Read the model definition and answer for the solid it produces. Units are mm, in the model's axes. Coordinates: 2 decimals unless noted, no trailing zeros.
1) Determine the mould class of faces 1 (the face through (-0.66, -14.985, 25.35)), 2 (the face through (4, -16, 0)) for opening direction X: +X half, -X half, draft (parallel to the pull), parting line (faces both ways), or undercut.
2) Each of these flat-tipped pins is pushed along its axis until it touches: pin 1 Ø2 at (y, z) = (-28.5, 39) entering from +X; pin 2 Ø12 at (x, z) = (-43.5, 10.5) entering from +Y; pin 3 Ø6 at (x, z) = (28.5, 42.5) entering from +Y. Where does it stop, or does it pass through?
3) Find the intervals of material crossed by line 1 (Y direction, x = 0, z = 38); line 2 (Y direction, x = 0, z = 24); line 3 (X direction, y = 1, z = 48.5), in increasing order.
Autodesk Inventor part; units mm, degrees
ref_plane "Work Plane1" through (0, 0, 50) normal (0, 0, 1) x (1, 0, 0)
ref_plane "YZ Plane" through (0, 0, 0) normal (1, 0, 0) x (0, 1, 0)
ref_plane "XZ Plane" through (0, 0, 0) normal (0, 1, 0) x (-1, 0, 0)
sketch "Sketch3" plane through (0, 0, 0) normal (0, 0, 1) x (1, 0, 0)
  line L0 (28.8675, 50) -> (57.735, 0)
  line L1 (57.735, 0) -> (28.8675, -50)
  line L2 (28.8675, -50) -> (-28.8675, -50)
  line L3 (-28.8675, -50) -> (-57.735, 0)
  line L4 (-57.735, 0) -> (-28.8675, 50)
  line L5 (-28.8675, 50) -> (28.8675, 50)
  point P0 (0, 0)
  point P1 (0, 50)
  dimension "DS_HEX_R1" = 50
ref_plane "Work Plane1" through (0, 0, 50) normal (0, 0, 1) x (1, 0, 0)
sketch "Sketch4" plane through (0, 0, 50) normal (0, 0, 1) x (1, 0, 0)
  line L0 (17.3205, 30) -> (34.641, 0)
  line L1 (34.641, 0) -> (17.3205, -30)
  line L2 (17.3205, -30) -> (-17.3205, -30)
  line L3 (-17.3205, -30) -> (-34.641, 0)
  line L4 (-34.641, 0) -> (-17.3205, 30)
  line L5 (-17.3205, 30) -> (17.3205, 30)
  point P0 (0, 0)
  point P1 (0, 0)
  point P2 (0, 30)
  dimension "d16" = 0
  dimension "DS_HEX_R2" = 30
loft "Loft1" add profiles "Sketch3", "Sketch4"
sketch "Sketch6" plane through (0, 0, 0) normal (0, 0, 1) x (1, 0, 0)
  point P0 (0, 0)
hole "Hole3" at (0, 0, 0) direction (0, 0, 1) diameter 30 end through all
properties part number "ai_param_dsdm_part1"
Reported:
1. face 1: undercut
1. face 2: draft
2. pin 1: stops at x = 24.01
2. pin 2: stops at y = 27.7
2. pin 3: stops at y = 22.36
3. line 1: y = -34.8 to -15, 15 to 34.8
3. line 2: y = -40.4 to -15, 15 to 40.4
3. line 3: x = -34.76 to -14.97, 14.97 to 34.76
